Build history of the part. All positions in model axes, mm. Face numbers are marked on the shaded views. A direction names the side the tool comes from. Round coordinates to 2 decimals unless told otherwise and drop trailing zeros. Write each loop counter-clockwise with the first axis right and the second up, starting at its lowest first coordinate (ties: lowest second). Pieces come first, ordered by that corner, then holes. Notation, with made-up numbers: M -21,0 L 9,0 A26 ccw 9,27 Z; hole C 80,29.5 d8. An arc over 180 degrees is marked long. Use a Markdown table: item, result.
from build123d import *

# Parameters (mm, degrees)
SKETCH10_R         = 2.291358881
CUT_EXTRUDE2_DEPTH = 2.0447
CUT_EXTRUDE2_DRAFT = -45
CUT_EXTRUDE1_DEPTH = 2.0447


with BuildPart() as part:
    # Sketch2 → Revolve1 (revolve)
    with BuildSketch(Plane(origin=(0, 0, 0), x_dir=(0, 0, -1), z_dir=(1, 0, 0))):
        Polygon((-12.618212, 6.7437), (-8.512892265, 3.175), (11.7475, 3.175), (12.7, 2.2225), (12.7, 0), (-12.7, 0), (-12.7, 6.7437), align=None)
    revolve(axis=Axis((0, 0, -12.7), (0, 0, 1)))


with BuildPart() as cut_extrude2_tool:
    # Sketch10 → Cut-Extrude2 (with draft: the straight prism first)
    with BuildSketch(Plane.XY.offset(12.7)):
        Circle(SKETCH10_R)
    extrude(amount=-CUT_EXTRUDE2_DEPTH)
    # Cut-Extrude2: the draft: its side faces are tilted about the plane it starts from
    cut_extrude2_sides = [cut_extrude2_tool.faces().sort_by_distance(p)[0] for p in [
        (-2.291358881, 0, 11.67765),
    ]]
    draft(cut_extrude2_sides, Plane.XY.offset(12.7), CUT_EXTRUDE2_DRAFT)


with BuildPart() as part_1:
    add(part.part)

    # Cut-Extrude2: cut by cut_extrude2_tool
    add(cut_extrude2_tool.part, mode=Mode.SUBTRACT)

    # Sketch9 → Cut-Extrude1 (cut)
    with BuildSketch(Plane.XY.offset(12.7)):
        Polygon((1.984375, -1.14567944), (1.984375, 1.14567944), (0, 2.291358881), (-1.984375, 1.14567944), (-1.984375, -1.14567944), (0, -2.291358881), align=None)
    extrude(amount=-CUT_EXTRUDE1_DEPTH, mode=Mode.SUBTRACT)


with BuildPart() as body_2:
    # Split1: the piece on the far side of the plane
    add(part_1.part)
    split(bisect_by=Plane.XY.offset(8.512892265), keep=Keep.BOTTOM)


with BuildPart() as part_2:
    add(part_1.part)

    # Split1
    split(bisect_by=Plane.XY.offset(8.512892265), keep=Keep.TOP)

    add(body_2.part)  # Boss-Extrude2 merges body 2
    # Boss-Extrude2 cone 1 section (through the dimple's axis) → Boss-Extrude2 (revolve)
    with BuildSketch(Plane(origin=(0, 0, 8.512892265), x_dir=(0, -1, 0), z_dir=(1, 0, 0))):
        Polygon((0, 0), (3.175, 0), (0, 8.723240807), align=None)
    revolve(axis=Axis((0, 0, 8.512892265), (0, 0, -1)))

    # Sketch12 → Cut-Revolve1 (revolve, cut)
    with BuildSketch(Plane(origin=(0, 0, 0), x_dir=(0, 0, -1), z_dir=(1, 0, 0))):
        with BuildLine():
            Line((-12.7, 0), (-12.7, 6.814797224))
            Line((-12.7, 6.814797224), (-11.988296252, 6.196122595))
            ThreePointArc((-11.988296252, 6.196122595), (-12.161061241, 6.221172326), (-12.2555, 6.074350831))
            Line((-12.2555, 6.074350831), (-12.2555, 0))
            Line((-12.2555, 0), (-12.7, 0))
        make_face()
    revolve(axis=Axis((0, 0, 0), (0, 0, 1)), mode=Mode.SUBTRACT)


solid = part_2.part
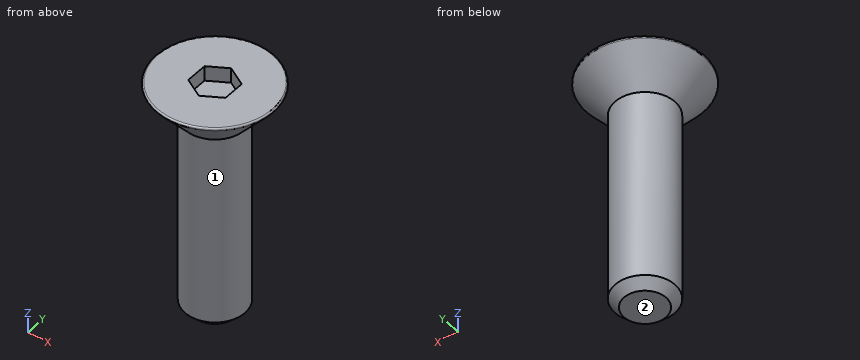
Q1. Which spindle directions (+Z, -Z, +X, -X, +Y, -Y) get a long thin tool onto all of the face, cutting with end or side? Do the marked faces 1 and 2. Say none if no direction does.
Response values:
| item | result |
|---|---|
| face 1 | -Z |
| face 2 | -Z, +X, -X, +Y, -Y |
Q2. Cut at C-C on z = 9. Give the cut face in (x, y).
Response values:
| item | result |
|---|---|
| outline | C 0,0 d7.2 |
Q3. Drill centre lines: L1, parallel to Z at x = -0.5, y = -1; L2, parallel to Z at x = -3.75, y = 2.75; L3, parallel to X at y = -0.5, z = -10. Where is each one in solid material? Low to high.
Response values:
| item | result |
|---|---|
| L1 | z = -12.7 to 10.66 |
| L2 | z = 10.21 to 12.26 |
| L3 | x = -3.14 to 3.14 |
Q4. Drop flat-ended pins along their axis: P1, Ø1.5, axis at x = -2.5, y = -2, coming from the -Z side; P2, Ø1.5, axis at y = 2, z = 9, coming from the +X side; P3, Ø4, axis at x = -1.5, z = 5.5, coming from the -Y side (3 decimals). Give the stop position or say it passes through.
Response values:
| item | result |
|---|---|
| P1 | stops at z = -12.47 |
| P2 | stops at x = 3.84 |
| P3 | stops at y = -3.175 |
Q5. Cut at B-B on z = -11. Give the cut face in (x, y) (3 decimals), and give its area (3 significant figures).
Response values:
| item | result |
|---|---|
| outline | C 0,0 d6.35 |
| area | 31.7 mm2 |
